```python
from build123d import *

# Parameters (mm, degrees)
SKETCH1_W                       = 100
SKETCH1_H                       = 100
BOSS_EXTRUDE1_DEPTH             = 50
M8X1_25_TAPPED_HOLE1_D          = 6.8
M8X1_25_TAPPED_HOLE1_DEPTH      = 27.75
M8X1_25_TAPPED_HOLE1_TIP        = 2.042926105
M8X1_0_TAPPED_HOLE1_D           = 7
M8X1_0_TAPPED_HOLE1_DEPTH       = 19
M8X1_0_TAPPED_HOLE1_TIP         = 2.103012167
M6X1_0_TAPPED_HOLE1_D           = 5
M6X1_0_TAPPED_HOLE1_DEPTH       = 15
M6X1_0_TAPPED_HOLE1_TIP         = 1.502151548
CBORE_FOR_M12_SHCS1_D           = 13.5
CBORE_FOR_M12_SHCS1_DEPTH       = 35
CBORE_FOR_M12_SHCS1_CBORE_D     = 20
CBORE_FOR_M12_SHCS1_CBORE_DEPTH = 12
CBORE_FOR_M12_SHCS1_TIP         = 4.055809178


with BuildPart() as part:
    # Sketch1 → Boss-Extrude1 (new body, symmetric)
    with BuildSketch(Plane.XY):
        Rectangle(SKETCH1_W, SKETCH1_H)
    extrude(amount=BOSS_EXTRUDE1_DEPTH, both=True)

    # M8x1.25 Tapped Hole1
    with Locations(Plane.ZY.offset(50)):
        with Locations((0, 0)):
            Hole(M8X1_25_TAPPED_HOLE1_D / 2, depth=M8X1_25_TAPPED_HOLE1_DEPTH)
            with Locations((0, 0, -(M8X1_25_TAPPED_HOLE1_DEPTH + M8X1_25_TAPPED_HOLE1_TIP / 2))):  # 118° drill point
                Cone(0, M8X1_25_TAPPED_HOLE1_D / 2, M8X1_25_TAPPED_HOLE1_TIP, mode=Mode.SUBTRACT)

    # M8x1.0 Tapped Hole1
    with Locations(Plane.XY.offset(50)):
        with Locations((0, 0)):
            Hole(M8X1_0_TAPPED_HOLE1_D / 2, depth=M8X1_0_TAPPED_HOLE1_DEPTH)
            with Locations((0, 0, -(M8X1_0_TAPPED_HOLE1_DEPTH + M8X1_0_TAPPED_HOLE1_TIP / 2))):  # 118° drill point
                Cone(0, M8X1_0_TAPPED_HOLE1_D / 2, M8X1_0_TAPPED_HOLE1_TIP, mode=Mode.SUBTRACT)

    # M6x1.0 Tapped Hole1
    with Locations(Plane(origin=(50, 0, 0), x_dir=(0, 0, -1), z_dir=(1, 0, 0))):
        with Locations((0, 0)):
            Hole(M6X1_0_TAPPED_HOLE1_D / 2, depth=M6X1_0_TAPPED_HOLE1_DEPTH)
            with Locations((0, 0, -(M6X1_0_TAPPED_HOLE1_DEPTH + M6X1_0_TAPPED_HOLE1_TIP / 2))):  # 118° drill point
                Cone(0, M6X1_0_TAPPED_HOLE1_D / 2, M6X1_0_TAPPED_HOLE1_TIP, mode=Mode.SUBTRACT)

    # CBORE for M12 SHCS1
    with Locations(Plane(origin=(0, 0, -50), x_dir=(-1, 0, 0), z_dir=(0, 0, -1))):
        with Locations((0, 0)):
            CounterBoreHole(CBORE_FOR_M12_SHCS1_D / 2, CBORE_FOR_M12_SHCS1_CBORE_D / 2, CBORE_FOR_M12_SHCS1_CBORE_DEPTH, depth=CBORE_FOR_M12_SHCS1_DEPTH)
            with Locations((0, 0, -(CBORE_FOR_M12_SHCS1_DEPTH + CBORE_FOR_M12_SHCS1_TIP / 2))):  # 118° drill point
                Cone(0, CBORE_FOR_M12_SHCS1_D / 2, CBORE_FOR_M12_SHCS1_TIP, mode=Mode.SUBTRACT)


solid = part.part
```
CAD build for the part. Positions are in the model's coordinates, mm. A direction names the side the tool comes from. Coordinates: 2 decimals unless noted, no trailing zeros.
(1) Two-plate mould, pull along X, no slides. Class faces 4 (the face through (2.17, -9.76, -44.08)), 5 (the face through (-1, 50, 1)), 6 (the face through (-50, -1, 12)): +X half, -X half, draft (parallel to the pull), parting line (faces both ways), or undercut.
(2) 3-axis set-ups, long thin cutter, end or side, ignore diameter. For faces 1 (the face through (-35.93, -3.32, 0.74)), 2 (the face through (-3.233, -1.341, 40.367)), 3 (the face through (-7, -2, -38)): which of +Z, -Z, +X, -X, +Y, -Y reach the whole face in a straight line?
(3) Flat gauge pins, fed straight in: pin 1 (10 mm diameter, centred on x = -2.5, y = 1.5, fed in from -Z); pin 2 (6.5 mm diameter, centred on y = 0, z = 0, fed in from -X); pin 3 (6.5 mm diameter, centred on x = 0, y = 0, fed in from -Z). Where does each tip first touch, or does it go through?
(4) Drill centre lines: probe 1 along Y at (x, z) = (0, 35); probe 2 along Y at (x, z) = (0, -46); probe 3 along Z at (x, y) = (40, -1). Where is each one in solid material? Low to high.
Geometry says:
1. face 4: undercut
1. face 5: draft
1. face 6: -X half
2. face 1: -X
2. face 2: +Z
2. face 3: -Z
3. pin 1: stops at z = -38
3. pin 2: stops at x = -22.16
3. pin 3: stops at z = -12.9
4. probe 1: y = -50 to -3.5, 3.5 to 50
4. probe 2: y = -50 to -10, 10 to 50
4. probe 3: z = -50 to -2.29, 2.29 to 50
